Here's how the part is built. I have some questions about the finished solid (model axes, mm). Face numbers are marked on the shaded views. A direction names the side the tool comes from. Round coordinates to 2 decimals unless told otherwise and drop trailing zeros. Order: outer loops, then holes, each group sorted by start corner. A loop starts at its lowest first (then second) coordinate and runs counter-clockwise, first axis right, second up. Notation, with made-up numbers: M 83,39 L 104,39 A8 ccw 104,53 Z; hole C -21,64 d1. An arc over 180 degrees is marked long. Write each question's results on one line, items separated by ' | '. Start each with the question number.
```python
from build123d import *

# Parameters (mm, degrees)
BOSS_EXTRUDE1_DEPTH = 5
SKETCH2_R           = 1.7
CUT_EXTRUDE1_DEPTH  = 28.386127875
SKETCH5_W           = 3
SKETCH5_H           = 4
SKETCH5_H_2         = 3.869300193
BOSS_EXTRUDE2_DEPTH = 10
SKETCH7_R           = 1.7
CUT_EXTRUDE2_DEPTH  = 31.822070015


with BuildPart() as part:
    # Sketch1 → Boss-Extrude1 (new body)
    with BuildSketch(Plane(origin=(0, 0, 0), x_dir=(0, 1, 0), z_dir=(0, 0, 1))):
        with BuildLine():
            Line((0, 0), (25, 0))
            Line((25, 0), (25, 3))
            Line((25, 3), (16.193237063, 3))
            ThreePointArc((16.193237063, 3), (8.3, 5), (16.193237063, 7))
            Line((16.193237063, 7), (25, 7))
            Line((25, 7), (25, 10))
            Line((25, 10), (0, 10))
            ThreePointArc((0, 10), (-5, 5), (0, 0))
        make_face()
    boss_extrude1 = extrude(amount=BOSS_EXTRUDE1_DEPTH)

    # Sketch2 → Cut-Extrude1 (cut, through all)
    with BuildSketch(Plane.XY.offset(5)):
        with Locations((-5, 0)):
            Circle(SKETCH2_R)
    extrude(amount=-CUT_EXTRUDE1_DEPTH, mode=Mode.SUBTRACT)

    # Sketch5 → Boss-Extrude2 (add)
    with BuildSketch(Plane.XY.offset(15)):
        with Locations((-8.5, 23)):
            Rectangle(SKETCH5_W, SKETCH5_H)
        with Locations((-1.5, 23.065349903)):
            Rectangle(SKETCH5_W, SKETCH5_H_2)
    extrude(amount=-BOSS_EXTRUDE2_DEPTH)

    # Mirror2: Boss-Extrude1 across plane
    add(boss_extrude1.mirror(Plane.XY.offset(7.5)))

    # Sketch7 → Cut-Extrude2 (cut, through all)
    with BuildSketch(Plane.XY.offset(15)):
        with Locations((-5, 0)):
            Circle(SKETCH7_R)
    extrude(amount=-CUT_EXTRUDE2_DEPTH, mode=Mode.SUBTRACT)


solid = part.part
```
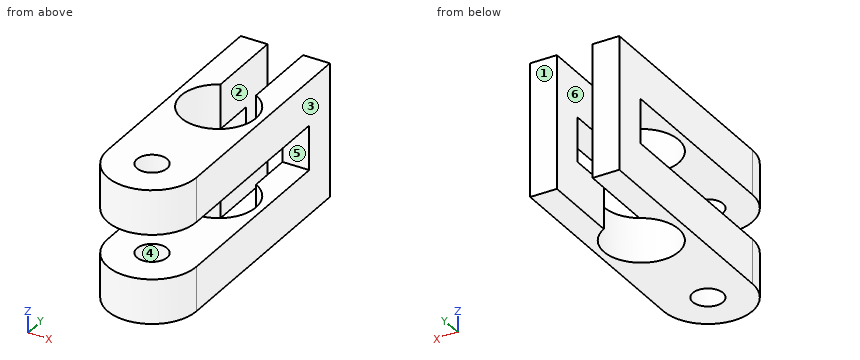
(1) Please list where these lines run through material, in increasing order: line 1 (Y direction, x = -5, z = 12.65); line 2 (Z direction, x = -1.75, y = 5); line 3 (X direction, y = 12.5, z = 2.8).
(2) If we mould it in two halves opening along X, with no side actions, what happens to the marked faces 1, 2 and 3? For each: pulls with the +X half, pulls with the -X half, needs draft (parallel to the pull), parting line crosses it, or undercut.
(3) I want a section at D-D on z = 11.5. Write out the boundary of the cut face in (x, y).
(4) I want a section at B-B on z = 7.25. Write out the boundary of the cut face in (x, y), and give its area (3 significant figures).
(5) I want a section at C-C on x = -5. Write out the boundary of the cut face in (y, z).
(6) On a 3-axis mill with a long thin cutter (end or side, diameter ignored), from which of +Z, -Z, +X, -X, +Y, -Y can I reach the whole of each face in a straight line? I mean the marked faces 4, 5 and 6. Say none if no direction works.
(7) I'm going to push flat-ended pins straight in: pin 1 Ø3 at (y, z) = (19, 5.5) entering from +X; pin 2 Ø3 at (x, z) = (-2, 6) entering from -Y; pin 3 Ø3.5 at (x, z) = (-1, 7) entering from -Y; pin 4 Ø3.5 at (x, z) = (-9, 7.5) entering from -Y. Where does each tip first touch, or does it pass through?
(8) I want a section at A-A on y = 12.5. Write out the boundary of the cut face in (x, z), and give its area (3 significant figures).
Solutions:
1) line 1: -5 to -1.7, 1.7 to 8.3 | line 2: 0 to 5, 10 to 15 | line 3: -10 to -9.2, -0.8 to 0
2) face 1: needs draft | face 2: undercut | face 3: pulls with the +X half
3) outline: M -10,0 A5 ccw 0,0 L 0,25 L -3,25 L -3,16.19 A4.2 cw long -7,16.19 L -7,25 L -10,25 Z; hole C -5,0 d3.4
4) outline: M -10,21 L -7,21 L -7,25 L -10,25 Z; M -3,21.13 L 0,21.13 L 0,25 L -3,25 Z | area: 23.6 mm^2
5) outline: M -5,0 L -1.7,0 L -1.7,5 L -5,5 Z; M -5,10 L -1.7,10 L -1.7,15 L -5,15 Z; M 1.7,0 L 8.3,0 L 8.3,5 L 1.7,5 Z; M 1.7,10 L 8.3,10 L 8.3,15 L 1.7,15 Z
6) face 4: +Z, -Z | face 5: +X, -Y | face 6: +Z, -Z, +Y
7) pin 1: x = 0 | pin 2: y = -4.63 | pin 3: y = 21.13 | pin 4: y = 21
8) outline: M -10,0 L -9.2,0 L -9.2,5 L -10,5 Z; M -10,10 L -9.2,10 L -9.2,15 L -10,15 Z; M -0.8,0 L 0,0 L 0,5 L -0.8,5 Z; M -0.8,10 L 0,10 L 0,15 L -0.8,15 Z | area: 16.0 mm^2
